Build history of the part. All positions in model axes, mm. Face numbers are marked on the shaded views. Coordinates: 2 decimals unless noted, no trailing zeros. Write each loop counter-clockwise with the first axis right and the second up, starting at its lowest first coordinate (ties: lowest second). Pieces come first, ordered by that corner, then holes.
```python
from build123d import *

# Parameters (mm, degrees)
F1_DEPTH  = 406
F4_DEPTH  = 22
F7_DEPTH  = 22
F9_W      = 350
F9_H      = 310
F10_DEPTH = 200


# Not quite as in the source:
# - ends of sketch curves that miss each other by under 0.0002 mm in the source are joined


with BuildPart() as f1:
    # F0 (on Front) → F1 (new body)
    with BuildSketch(Plane.XZ):
        with BuildLine():
            ThreePointArc((-186.3848490661, -11.1654008205), (33.2859089962, 22.935224068), (249.0237497892, -30.686400445))
            Line((249.0237497892, -30.686400445), (253.556713, -20.661948))
            ThreePointArc((253.556713, -20.661948), (33.6810541326, 33.9285497238), (-190.1858030941, -0.8429617445))
            Line((-190.1858030941, -0.8429617445), (-253.556714, -24.177561))
            Line((-253.556714, -24.177561), (-249.755724, -34.499987))
            Line((-249.755724, -34.499987), (-186.3848490661, -11.1654008205))
        make_face()
    extrude(amount=F1_DEPTH)

    # F3 (on offset) → F4 (cut)
    with BuildSketch(Plane.XZ.offset(395)):
        with BuildLine():
            Line((184.0178133859, -9.9744413883), (190.6417317828, 9.9535215049))
            ThreePointArc((190.6417317828, 9.9535215049), (-1.1548935515, 39.4263138769), (-191.9135098522, 3.8490558767))
            Line((-191.9135098522, 3.8490558767), (-184.6571423005, -15.8574184389))
            ThreePointArc((-184.6571423005, -15.8574184389), (-0.819837913, 18.4289869585), (184.0178133859, -9.9744413883))
        make_face()
    extrude(amount=-F4_DEPTH, mode=Mode.SUBTRACT)

    # F6 (on offset) → F7 (cut)
    with BuildSketch(Plane(origin=(0, -11, 0), x_dir=(-1, 0, 0), z_dir=(0, 1, 0))):
        with BuildLine():
            ThreePointArc((191.9135098522, 3.8490558767), (1.1548935515, 39.4263138769), (-190.6417317828, 9.9535215049))
            Line((-190.6417317828, 9.9535215049), (-184.0178133859, -9.9744413883))
            ThreePointArc((-184.0178133859, -9.9744413883), (0.819837913, 18.4289869585), (184.6571423005, -15.8574184389))
            Line((184.6571423005, -15.8574184389), (191.9135098522, 3.8490558767))
        make_face()
    extrude(amount=-F7_DEPTH, mode=Mode.SUBTRACT)

    # F9 (on offset) → F10 (cut)
    with BuildSketch(Plane.XY.offset(134)):
        with Locations((-5e-07, -203)):
            Rectangle(F9_W, F9_H)
    extrude(amount=-F10_DEPTH, mode=Mode.SUBTRACT)


solid = f1.part
```
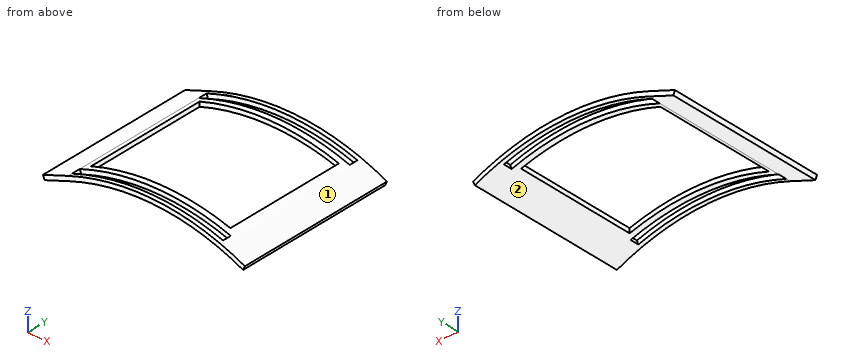
1. Probe line 1 along Y through (x, z) = (-153, 6); line 2 along Z through (x, y) = (-179.5, -359); line 3 along Z through (x, y) = (-214, -155.5). List the from-to ranges inside material, lowest first.
Computed values:
line 1: y = -406 to -395, -373 to -358, -48 to -33, -11 to 0
line 2: z = -8.68 to 2.97
line 3: z = -21.33 to -9.61
2. Saw through at C-C on x = 146. List the corners of the cut face in (y, z).
Computed values:
outline: (-406, 6.34) - (-395, 6.34) - (-395, 17.68) - (-406, 17.68) - close; (-373, 6.34) - (-358, 6.34) - (-358, 17.68) - (-373, 17.68) - close; (-48, 6.34) - (-33, 6.34) - (-33, 17.68) - (-48, 17.68) - close; (-11, 6.34) - (0, 6.34) - (0, 17.68) - (-11, 17.68) - close
3. Mould opens along X. For the marked faces 1 and 2 say: +X half, -X half, draft (parallel to the pull), parting line (faces both ways), or undercut.
Computed values:
face 1: parting line
face 2: undercut
4. Saw through at A-A on y = -318. List the corners of the cut face in (x, z).
Computed values:
outline: (-253.56, -24.18) - (-249.76, -34.5) - (-186.38, -11.17) arc R562.78 cw to (-175, -7.11) - (-175, 4.51) arc R573.78 ccw to (-190.19, -0.84) - close; (175, -1.82) arc R562.78 cw to (249.02, -30.69) - (253.56, -20.66) arc R573.78 ccw to (175, 9.68) - close
5. Flat gauge pins, fed straight in: pin 1 (5 mm diameter, centred on y = -210.5, z = -22, fed in from -X); pin 2 (5 mm diameter, centred on y = -67.5, z = 8.5, fed in from -X). Where does each tip first touch, or does it go through?
Computed values:
pin 1: stops at x = -253.56
pin 2: stops at x = 175
6. Saw through at D-D on y = -38.5. List the corners of the cut face in (x, z).
Computed values:
outline: (-253.56, -24.18) - (-249.76, -34.5) - (-186.38, -11.17) arc R562.78 cw to (249.02, -30.69) - (253.56, -20.66) arc R573.78 ccw to (-190.19, -0.84) - close
7. Saw through at B-B on x = -86. List the corners of the cut face in (y, z), plus the area to 3 significant figures.
Computed values:
outline: (-406, 15.58) - (-395, 15.58) - (-395, 26.73) - (-406, 26.73) - close; (-373, 15.58) - (-358, 15.58) - (-358, 26.73) - (-373, 26.73) - close; (-48, 15.58) - (-33, 15.58) - (-33, 26.73) - (-48, 26.73) - close; (-11, 15.58) - (0, 15.58) - (0, 26.73) - (-11, 26.73) - close
area: 580 mm2
